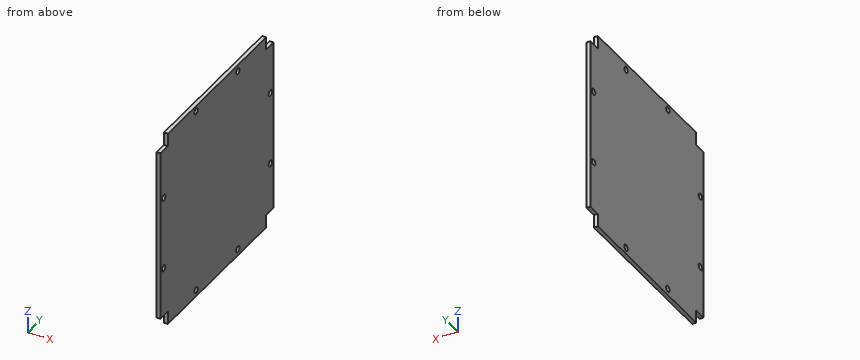
Autodesk Fusion 360 part; units mm, degrees
sketch "Sketch1" plane through (0, 0, 0) normal (1, 0, 0) x (0, 0, -1)
  line L0 (0, 0) -> (-100, 0)
  line L1 (-100, 0) -> (-100, 100)
  line L2 (-100, 100) -> (0, 100)
  line L3 (0, 100) -> (0, 0)
  dimension "d1" = 100
  dimension "d2" = 100
extrude "Extrude1" add sketch "Sketch1" against normal blind 2
extrude "Extrude2" add 1 faces at (0, 33.3333, 33.3333) along direction (1, 0, 0) blind 2
extrude "Extrude3" add 1 faces at (2, 33.3333, 33.3333) along direction (1, 0, 0) blind 1
sketch "Sketch2" plane through (3, 0, 0) normal (1, 0, 0) x (0, 0, -1)
  line L0 (-100, 100) -> (0, 100)
  line L1 (0, 100) -> (0, 0)
  line L2 (0, 0) -> (-100, 0)
  line L3 (-100, 0) -> (-100, 100)
  line L4 (-100, 100) -> (-68.5, 100)
  line L5 (-68.5, 100) -> (-68.5, 94.5)
  line L6 (-68.5, 94.5) -> (-100, 94.5)
  line L7 (-100, 94.5) -> (-100, 100)
  line L8 (-100, 100) -> (-93.5, 100)
  line L9 (-93.5, 100) -> (-93.5, 68.5)
  line L10 (0, 100) -> (-6.5, 100)
  line L11 (-6.5, 100) -> (-6.5, 68.5)
  line L12 (-6.5, 68.5) -> (0, 68.5)
  line L13 (0, 68.5) -> (0, 100)
  line L14 (0, 100) -> (-31.5, 100)
  line L15 (-31.5, 100) -> (-31.5, 94.5)
  line L16 (-31.5, 94.5) -> (0, 94.5)
  line L17 (0, 94.5) -> (0, 100)
  line L18 (0, 0) -> (-6.5, 0)
  line L19 (-6.5, 0) -> (-6.5, 31.5)
  line L20 (-6.5, 31.5) -> (0, 31.5)
  line L21 (0, 31.5) -> (0, 0)
  line L22 (0, 0) -> (-31.5, 0)
  line L23 (-31.5, 0) -> (-31.5, 5.5)
  line L24 (-31.5, 5.5) -> (0, 5.5)
  line L25 (0, 5.5) -> (0, 0)
  line L26 (-100, 0) -> (-68.5, 0)
  line L27 (-68.5, 0) -> (-68.5, 5.5)
  line L28 (-68.5, 5.5) -> (-100, 5.5)
  line L29 (-100, 5.5) -> (-100, 0)
  line L30 (-100, 0) -> (-94.5, 0)
  line L31 (-94.5, 0) -> (-94.5, 31.5)
  line L32 (-94.5, 31.5) -> (-100, 31.5)
  line L33 (-100, 31.5) -> (-100, 0)
  circle A0 centre (-68.5, 97.25) radius 1.5
  circle A1 centre (-97.25, 31.5) radius 1.5
  circle A2 centre (-68.5, 2.75) radius 1.5
  circle A3 centre (-31.5, 2.75) radius 1.5
  circle A4 centre (-3.25, 31.5) radius 1.5
  circle A5 centre (-3.25, 68.5) radius 1.5
  circle A6 centre (-31.5, 97.25) radius 1.5
  line L34 (-93.5, 68.5) -> (-100, 68.5)
  line L35 (-100, 68.5) -> (-100, 100)
  line L36 (-100, 100) -> (-93.5, 100)
  line L37 (-93.5, 100) -> (-93.5, 68.5)
  circle A7 centre (-96.75, 68.5) radius 1.5
  line L38 (-100, 100) -> (-93.5, 100)
  line L39 (-93.5, 100) -> (-93.5, 93.5)
  line L40 (-93.5, 93.5) -> (-100, 93.5)
  line L41 (-100, 93.5) -> (-100, 100)
  line L42 (-100, 0) -> (-93.5, 0)
  line L43 (-93.5, 0) -> (-93.5, 6.5)
  line L44 (-93.5, 6.5) -> (-100, 6.5)
  line L45 (-100, 6.5) -> (-100, 0)
  line L46 (0, 0) -> (-6.5, 0)
  line L47 (-6.5, 0) -> (-6.5, 6.5)
  line L48 (-6.5, 6.5) -> (0, 6.5)
  line L49 (0, 6.5) -> (0, 0)
  line L50 (0, 100) -> (-6.5, 100)
  line L51 (-6.5, 100) -> (-6.5, 93.5)
  line L52 (-6.5, 93.5) -> (0, 93.5)
  line L53 (0, 93.5) -> (0, 100)
  dimension "d53" = 31.5
  dimension "d54" = 5.5
  dimension "d55" = 6.5
  dimension "d57" = 6.5
  dimension "d58" = 31.5
  dimension "d59" = 31.5
  dimension "d60" = 5.5
  dimension "d61" = 6.5
  dimension "d62" = 31.5
  dimension "d63" = 5.5
  dimension "d64" = 31.5
  dimension "d65" = 5.5
  dimension "d66" = 31.5
  dimension "d67" = 100
  dimension "d68" = 100
  dimension "d69" = 5.5
  dimension "d70" = 31.5
  dimension "d71" = 3
  dimension "d73" = 3
  dimension "d74" = 3
  dimension "d75" = 3
  dimension "d76" = 3
  dimension "d77" = 3
  dimension "d78" = 3
  dimension "d81" = 31.5
  dimension "d83" = 3
  dimension "d88" = 6.5
  dimension "d89" = 6.5
  dimension "d90" = 6.5
  dimension "d91" = 6.5
  dimension "d92" = 6.5
  dimension "d93" = 6.5
  dimension "d94" = 6.5
  dimension "d95" = 6.5
extrude "Extrude9" cut sketch "Sketch2" against normal blind 20 contours L5 A0 | L5 A0 | L15 A6 | L15 A6 | L34 A7 | L34 A7 | L32 A1 | L32 A1 | L12 A5 | L12 A5 | L20 A4 | L20 A4 | L27 A2 | L27 A2 | L23 A3 | L23 A3
extrude "Extrude10" cut sketch "Sketch2" against normal blind 3 contours L0 L3 L4 L6 L7 L8 L9 L35 L36 L37 L38 L39 L41 | L0 L4 L5 L6 L9 A0 L37 L39 | L3 L6 L9 L35 L37 L39 L40 L41 | L0 L1 L2 L3 L5 L6 L9 L11 L12 L15 L16 L19 L20 L23 L24 L27 L28 L31 L32 A0 A1 A2 A3 A4 A5 A6 L34 L37 A7 L39 L43 L44 L47 L51 | L3 L9 L34 L35 L37 A7 L40 | L0 L11 L14 L15 L16 A6 L51 | L0 L1 L10 L11 L13 L14 L16 L17 L50 L51 L53 | L3 L31 L32 L33 A1 L44 | L1 L11 L13 L16 L51 L52 L53 | L3 L28 L31 L33 L44 L45 | L1 L11 L12 L13 A5 L52 | L2 L3 L26 L28 L29 L30 L31 L33 L42 L45 | L28 L31 L43 L44 | L2 L26 L28 L31 L42 L43 | L2 L26 L27 L28 A2 L43 | L1 L19 L20 L21 A4 L48 | L1 L19 L21 L24 L47 L48 L49 | L1 L2 L18 L19 L21 L22 L24 L25 L46 L47 L49 | L2 L19 L22 L23 L24 A3 L47
extrude "Extrude11" cut sketch "Sketch2" against normal blind 70 contours L0 L3 L4 L6 L7 L8 L9 L35 L36 L37 L38 L39 L41 | L3 L6 L9 L35 L37 L39 L40 L41 | L0 L1 L10 L11 L13 L14 L16 L17 L50 L51 L53 | L1 L11 L13 L16 L51 L52 L53 | L3 L28 L31 L33 L44 L45 | L2 L3 L26 L28 L29 L30 L31 L33 L42 L45 | L28 L31 L43 L44 | L2 L26 L28 L31 L42 L43 | L1 L19 L21 L24 L47 L48 L49 | L1 L2 L18 L19 L21 L22 L24 L25 L46 L47 L49
Input: part model. Units: mm. Frame: model coordinates. Coordinates: 2 decimals unless noted, no trailing zeros. Loops run counter-clockwise (first coordinate to the right, second up) from the corner with the lowest first, then second, coordinate; pieces in that order, holes last.
Q1. Contact query for flat-ended pins moving along their axis: pin 1 (1 mm diameter, centred on x = -1, y = 96.5, fed in from +Z); pin 2 (0.6 mm diameter, centred on x = -0.5, y = 3, fed in from -Z); pin 3 (0.6 mm diameter, centred on x = -1.5, z = 96.5, fed in from -Y). Output: stop coordinate, or through.
Results are:
pin 1: stops at z = 93.5
pin 2: stops at z = 6.5
pin 3: stops at y = 6.5
Q2. Line query: line 1 along Z through (x, y) = (-0.65, 68.5); line 2 along Y through (x, z) = (-1.15, 3.25); line 3 along Y through (x, z) = (-0.75, 68.5). Output: solid intervals per line, ascending.
Results are:
line 1: z = 0 to 1.75, 4.75 to 95.25, 98.25 to 100
line 2: y = 6.5 to 30, 33 to 67, 70 to 93.5
line 3: y = 0 to 1.25, 4.25 to 95.75, 98.75 to 100
Q3. Section C-C, the plane x = -1.35. Give the number of separate pieces and of enclosed holes in the cut face, and give its area (3 significant figures).
Results are:
separate pieces: 1
enclosed holes: 8
area: 9,770 mm2
Q4. Section B-B, the plane z = 3.25. Return the cut outline in (x, y), and give its area (3 significant figures).
Results are:
outline: (-2, 6.5) - (0, 6.5) - (0, 30) - (-2, 30) - close; (-2, 33) - (0, 33) - (0, 67) - (-2, 67) - close; (-2, 70) - (0, 70) - (0, 93.5) - (-2, 93.5) - close
area: 162 mm2
Q5. Section A-A, the plane y = 68.5. Return the cut outline in (x, z), and give its area (3 significant figures).
Results are:
outline: (-2, 0) - (0, 0) - (0, 1.75) - (-2, 1.75) - close; (-2, 4.75) - (0, 4.75) - (0, 95.25) - (-2, 95.25) - close; (-2, 98.25) - (0, 98.25) - (0, 100) - (-2, 100) - close
area: 188 mm2
